Check sheet for the modelled part. Datum: model origin and axes. Units: mm. Face numbers are marked on the shaded views. A direction names the side the tool comes from. Give positions to 0.01 mm unless a question says otherwise; leave off trailing zeros. Order: outer loops, then holes, each group sorted by start corner. A loop starts at its lowest first (then second) coordinate and runs counter-clockwise, first axis right, second up.
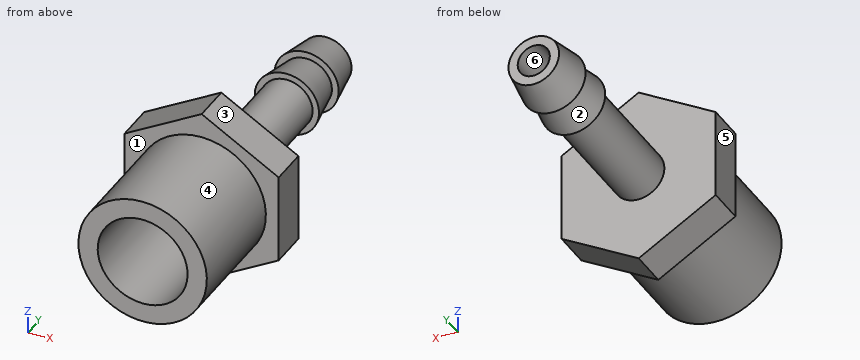
```python
from build123d import *

# Parameters (mm, degrees)
EXTRUSION1_DEPTH  = 3
ESQUISSE3_R       = 5
ESQUISSE3_R_2     = 3.5
EXTRUSION2_DEPTH  = 9
ESQUISSE4_R       = 2
EXTRUSION3_DEPTH  = 10
ESQUISSE5_R       = 2.5
EXTRUSION4_DEPTH  = 3
CHANFREIN1_SIZE   = 3
CHANFREIN1_SIZE_2 = 0.528980942
ESQUISSE6_R       = 2.5
EXTRUSION5_DEPTH  = 3
CHANFREIN2_SIZE   = 3
CHANFREIN2_SIZE_2 = 0.528980942
EXTRUSION6_REACH  = 31.462
ESQUISSE7_R       = 1.25


with BuildPart() as part:
    # Esquisse2 → Extrusion1 (new body)
    with BuildSketch(Plane(origin=(0, 0, 0), x_dir=(1, 0, 0), z_dir=(0, 1, 0))):
        Polygon((0, 6.92820323), (-6, 3.464101615), (-6, -3.464101615), (0, -6.92820323), (6, -3.464101615), (6, 3.464101615), align=None)
    extrude(amount=EXTRUSION1_DEPTH)

    # Esquisse3 → Extrusion2 (add)
    with BuildSketch(Plane.XZ):
        with Locations(Location((0, 0, 0), (0, 0, 90))):
            Circle(ESQUISSE3_R)
        with Locations(Location((0, 0, 0), (0, 0, 270))):
            Circle(ESQUISSE3_R_2, mode=Mode.SUBTRACT)
    extrude(amount=EXTRUSION2_DEPTH)

    # Esquisse4 → Extrusion3 (add)
    with BuildSketch(Plane(origin=(0, 3, 0), x_dir=(-1, 0, 0), z_dir=(0, 1, 0))):
        with Locations(Location((0, 0, 0), (0, 0, 90))):
            Circle(ESQUISSE4_R)
    extrude(amount=EXTRUSION3_DEPTH)

    # Esquisse5 → Extrusion4 (add)
    with BuildSketch(Plane(origin=(0, 13, 0), x_dir=(1, 0, 0), z_dir=(0, 1, 0))):
        with Locations(Location((0, 0, 0), (0, 0, 270))):
            Circle(ESQUISSE5_R)
    extrude(amount=EXTRUSION4_DEPTH)

    # Chanfrein1
    # the kernel refuses this chamfer: 3, 0.528980942 mm, written as the material it takes off along each edge
    with BuildSketch(Plane(origin=(0, 16, 0), x_dir=(0, 0, 1), z_dir=(-1, 0, 0))) as chanfrein1_piece_1:
        Polygon((2.5, -CHANFREIN1_SIZE), (2.5 - CHANFREIN1_SIZE_2, 0), (2.5, 0), align=None)
    revolve(axis=Axis((0, 16, 0), (0, 1, 0)), mode=Mode.SUBTRACT)

    # Esquisse6 → Extrusion5 (add)
    with BuildSketch(Plane(origin=(0, 16, 0), x_dir=(1, 0, 0), z_dir=(0, 1, 0))):
        with Locations(Location((0, 0, 0), (0, 0, 270))):
            Circle(ESQUISSE6_R)
    extrude(amount=EXTRUSION5_DEPTH)

    # Chanfrein2
    # the kernel refuses this chamfer: 3, 0.528980942 mm, written as the material it takes off along each edge
    with BuildSketch(Plane(origin=(0, 19, 0), x_dir=(0, 0, 1), z_dir=(-1, 0, 0))) as chanfrein2_piece_1:
        Polygon((2.5, -CHANFREIN2_SIZE), (2.5 - CHANFREIN2_SIZE_2, 0), (2.5, 0), align=None)
    revolve(axis=Axis((0, 19, 0), (0, 1, 0)), mode=Mode.SUBTRACT)

    # Esquisse7 → Extrusion6 (cut, up to next)
    with BuildSketch(Plane(origin=(0, 19, 0), x_dir=(1, 0, 0), z_dir=(0, 1, 0)), mode=Mode.PRIVATE) as extrusion6_sk1:
        with Locations(Location((0, 0, 0), (0, 0, 270))):
            Circle(ESQUISSE7_R)
    extrusion6_tool1 = extrude(extrusion6_sk1.sketch, amount=-EXTRUSION6_REACH, mode=Mode.PRIVATE) & part.part
    add(extrusion6_tool1.solids().sort_by_distance((0, 19, 0))[0], mode=Mode.SUBTRACT)


solid = part.part
```
(1) Cross-section at D-D on y = -2. Enter the section's corners in (x, z), then the cut area to 3 significant figures.
Response values:
outline: circle Ø10 at (0, 0); hole circle Ø7 at (0, 0)
area: 40.1 mm2
(2) Gauge pin test, flat ends, axial feed: pin 1 Ø6 at (x, y) = (2, 9) entering from -Z; pin 2 Ø6 at (x, z) = (-1, 0) entering from -Y; pin 3 Ø5 at (x, y) = (0.5, 12.5) entering from -Z; pin 4 Ø4 at (x, z) = (1, 1) entering from -Y. Record the tip position at first contact, or that the pin passes through.
Response values:
pin 1: stops at z = -2
pin 2: stops at y = -9
pin 3: stops at z = -2.5
pin 4: stops at y = 0
(3) Cross-section at A-A on z = 0. Enter the section's corners in (x, y).
Response values:
outline: (-6, 0) - (-5, 0) - (-5, -9) - (-3.5, -9) - (-3.5, 0) - (-1.25, 0) - (-1.25, 19) - (-1.97, 19) - (-2.5, 16) - (-1.97, 16) - (-2.5, 13) - (-2, 13) - (-2, 3) - (-6, 3) - close; (1.25, 0) - (3.5, 0) - (3.5, -9) - (5, -9) - (5, 0) - (6, 0) - (6, 3) - (2, 3) - (2, 13) - (2.5, 13) - (1.97, 16) - (2.5, 16) - (1.97, 19) - (1.25, 19) - close
(4) Set-up check for the marked faces 1, 2 and 3: record each of +Z, -Z, +X, -X, +Y, -Y from which the full face is reachable in a straight line by a thin tool's end or side.
Response values:
face 1: -Y
face 2: none
face 3: +Z, +X, +Y, -Y
(5) Cross-section at B-B on y = 1.75. Enter the section's corners in (x, z), then the cut area to 3 significant figures.
Response values:
outline: (-6, -3.46) - (0, -6.93) - (6, -3.46) - (6, 3.46) - (0, 6.93) - (-6, 3.46) - close; hole circle Ø2.5 at (0, 0)
area: 120 mm2
(6) Material ranges on L1, parallel to X at y = 5.5, z = 0; L2, parallel to X at y = -2.5, z = 0; L3, parallel to Y at x = -3.5, z = 3, recorded low to high.
Response values:
L1: x = -2 to -1.25, 1.25 to 2
L2: x = -5 to -3.5, 3.5 to 5
L3: y = -9 to 3
(7) Cross-section at C-C on x = -4.25. Enter the section's corners in (y, z), then the cut area to 3 significant figures.
Response values:
outline: (-9, -2.63) - (0, -2.63) - (0, -4.47) - (3, -4.47) - (3, 4.47) - (0, 4.47) - (0, 2.63) - (-9, 2.63) - close
area: 74.3 mm2
(8) Release check for a two-part mould opening along X. For the marked faces 4, 5 and 6 record: released by +X, released by -X, zero draft, split by the parting line, or undercut.
Response values:
face 4: split by the parting line
face 5: released by -X
face 6: undercut
